```python
from build123d import *

# Parameters (mm, degrees)
SKETCH1_R           = 1.869394483
BOSS_EXTRUDE1_DEPTH = 4
BOSS_EXTRUDE2_START = 4.5
BOSS_EXTRUDE2_DEPTH = 4.5
BOSS_EXTRUDE3_START = 4
BOSS_EXTRUDE3_DEPTH = 4
BOSS_EXTRUDE4_START = -3
SKETCH6_R           = 1.25
BOSS_EXTRUDE4_DEPTH = 3


with BuildPart() as part:
    # Sketch1 → Boss-Extrude1 (new body)
    with BuildSketch(Plane.XY):
        with BuildLine():
            Line((21.403000099, -27.721654021), (29.301617843, -36.205200538))
            ThreePointArc((29.301617843, -36.205200538), (29.193506427, -39.233088823), (26.165618141, -39.124977407))
            Line((26.165618141, -39.124977407), (18.267000397, -30.64143089))
            ThreePointArc((18.267000397, -30.64143089), (18.375111813, -27.613542605), (21.403000099, -27.721654021))
        make_face()
        with Locations((19.835000248, -29.181542456)):
            Circle(SKETCH1_R, mode=Mode.SUBTRACT)
    extrude(amount=BOSS_EXTRUDE1_DEPTH)

    # Sketch2 → Boss-Extrude2 (add)
    with BuildSketch(Plane(origin=(0, 0, 0), x_dir=(-1, 0, 0), z_dir=(0, 0, -1)).offset(BOSS_EXTRUDE2_START)):
        with BuildLine():
            Line((-29.301617843, -36.205200538), (-26.904832103, -33.63092185))
            Line((-26.904832103, -33.63092185), (-23.768832401, -36.55069872))
            Line((-23.768832401, -36.55069872), (-26.165618141, -39.124977407))
            ThreePointArc((-26.165618141, -39.124977407), (-29.193506427, -39.233088823), (-29.301617843, -36.205200538))
        make_face()
    extrude(amount=-BOSS_EXTRUDE2_DEPTH)

    # Sketch3 → Boss-Extrude3 (add)
    with BuildSketch(Plane(origin=(0, 0, -4.5), x_dir=(-1, 0, 0), z_dir=(0, 0, -1)).offset(BOSS_EXTRUDE3_START)):
        with BuildLine():
            Line((-26.165618141, -39.124977407), (-23.768832401, -36.55069872))
            Line((-23.768832401, -36.55069872), (-18.267000397, -30.64143089))
            ThreePointArc((-18.267000397, -30.64143089), (-18.375111813, -27.613542605), (-21.403000099, -27.721654021))
            Line((-21.403000099, -27.721654021), (-26.904832103, -33.63092185))
            Line((-26.904832103, -33.63092185), (-29.301617843, -36.205200538))
            ThreePointArc((-29.301617843, -36.205200538), (-29.193506427, -39.233088823), (-26.165618141, -39.124977407))
        make_face()
    extrude(amount=-BOSS_EXTRUDE3_DEPTH)

    # Sketch6 → Boss-Extrude4 (add)
    with BuildSketch(Plane.XY.offset(4).offset(BOSS_EXTRUDE4_START)):
        with BuildLine():
            Line((37.749845774, -51.567070083), (26.165618141, -39.124977407))
            ThreePointArc((26.165618141, -39.124977407), (26.273729557, -36.097089122), (29.301617843, -36.205200538))
            Line((29.301617843, -36.205200538), (40.885845475, -48.647293214))
            ThreePointArc((40.885845475, -48.647293214), (40.777734059, -51.675181499), (37.749845774, -51.567070083))
        make_face()
        with Locations((39.317845624, -50.107181648)):
            Circle(SKETCH6_R, mode=Mode.SUBTRACT)
    extrude(amount=BOSS_EXTRUDE4_DEPTH)


solid = part.part
```
Read the model definition and answer for the solid it produces. Units are mm, in the model's axes. A direction names the side the tool comes from. Give positions to 0.01 mm unless a question says otherwise; leave off trailing zeros. Loops run counter-clockwise (first coordinate to the right, second up) from the corner with the lowest first, then second, coordinate; pieces in that order, holes last.
Item 1: The part is cut by section A-A (y = -30). Write down the section's boundary in (x, z).
Item 2: Each of these flat-tipped pins is pushed along its axis until it touches: pin 1 Ø3 at (x, z) = (22.5, -7) entering from -Y; pin 2 Ø1.5 at (x, y) = (39.32, -50.11) entering from -Z; pin 3 Ø6 at (y, z) = (-35, -7) entering from +X; pin 4 Ø4 at (x, z) = (23, -7) entering from -Y. Where does it stop, or does it pass through?
Item 3: The mould has two halves that part along X. Classify faces 6 (the cylindrical face through (39.155, -48.868, 2.479)), 7 (the cylindrical face through (18.341, -27.646, -6.528)), 8 (the flat face through (31, -40, 4)): released by +X, released by -X, zero draft, split by the parting line, or undercut.
Item 4: The part is cut by section D-D (y = -49.75). Write down the section's boundary in (x, z).
Item 5: Find the intervals of material crossed by line 1 along Z through (x, y) = (23, -30.25); line 2 along Z through (x, y) = (35.5, -44.5); line 3 along X through (y, z) = (-36.5, 1.25), in increasing order.
Item 6: The part is cut by section C-C (z = -7). Write down the section's boundary in (x, y) (3 decimals), and give its area (3 significant figures).
Item 7: For faces 1 (the flat face through (24, -33, -8.5)), 2 (the cylindrical face through (29.23, -39.2, -3.82)), 3 (the cylindrical face through (20.7, -30.84, 1.97)), 4 (the flat face through (22, -32, -4.5)), 5 (the cylindrical face through (40.812, -51.643, 2.479)), determine the directions among +Z, -Z, +X, -X, +Y, -Y from which every point of the face is accessible in a straight line to the end or side of a thin tool.
Item 8: The part is cut by section B-B (x = 38.5). Write down the section's boundary in (y, z), and give its area (3 significant figures).
Taken from the geometry:
1. outline: (17.86, -8.5) - (23.52, -8.5) - (23.52, -4.5) - (17.86, -4.5) - close; (17.86, 0) - (18.15, 0) - (18.15, 4) - (17.86, 4) - close; (21.52, 0) - (23.52, 0) - (23.52, 4) - (21.52, 4) - close
2. pin 1: stops at y = -36.8
2. pin 2: passes through
2. pin 3: stops at x = 29.88
2. pin 4: stops at y = -37.87
3. face 6: undercut
3. face 7: split by the parting line
3. face 8: zero draft
4. outline: (36.06, 1) - (38.12, 1) - (38.12, 4) - (36.06, 4) - close; (40.52, 1) - (41.43, 1) - (41.43, 4) - (40.52, 4) - close
5. line 1: z = -8.5 to -4.5, 0 to 4
5. line 2: z = 1 to 4
5. line 3: x = 23.72 to 29.58
6. outline: (18.267, -30.641) - (26.166, -39.125) arc R2.142 ccw to (29.302, -36.205) - (21.403, -27.722) arc R2.142 ccw to start
6. area: 64.1 mm2
7. face 1: -Z, +X, -X, +Y, -Y
7. face 2: -Z
7. face 3: +Z
7. face 4: -X, +Y
7. face 5: +Z, -Z
8. outline: (-52.09, 1) - (-51.05, 1) - (-51.05, 4) - (-52.09, 4) - close; (-49.16, 1) - (-46.08, 1) - (-46.08, 4) - (-49.16, 4) - close
8. area: 12.3 mm2
